```python
from build123d import *

# Parameters (mm, degrees)
BOSS_EXTRUDE1_DEPTH = 16.4
SKETCH3_R           = 4.85
CUT_EXTRUDE1_DEPTH  = 55.101495482


with BuildPart() as part:
    # Sketch1 → Revolve1 (revolve)
    with BuildSketch(Plane.XY, mode=Mode.PRIVATE) as revolve1_sk:
        Polygon((0, 51.4), (0, 0), (10.9, 0), (10.9, 3.8), (11.05, 3.8), (11.05, 20.1), (10.9, 20.1), (10.9, 22.1), (7.9, 22.1), (7.9, 24.4), (6.35, 24.4), (6.35, 34.8), (7.95, 34.8), (6.35, 39.6), (6.35, 44.2), (7.55, 44.2), (6.35, 48.4), (6.35, 51.4), align=None)
    revolve(revolve1_sk.sketch.rotate(Axis((0, 51.4, 0), (0, -1, 0)), 180), axis=Axis((0, 51.4, 0), (0, -1, 0)))

    # Sketch2 → Boss-Extrude1 (add)
    with BuildSketch(Plane(origin=(0, 20.1, 0), x_dir=(1, 0, 0), z_dir=(0, 1, 0))):
        Polygon((12.761813873, 0), (6.380906937, 11.052055013), (-6.380906937, 11.052055013), (-12.761813873, 0), (-6.380906937, -11.052055013), (6.380906937, -11.052055013), align=None)
    extrude(amount=-BOSS_EXTRUDE1_DEPTH)

    # Sketch3 → Cut-Extrude1 (cut, through all)
    with BuildSketch(Plane(origin=(0, 51.4, 0), x_dir=(1, 0, 0), z_dir=(0, 1, 0))):
        with Locations(Location((0, 0, 0), (0, 0, 180))):
            Circle(SKETCH3_R)
    extrude(amount=-CUT_EXTRUDE1_DEPTH, mode=Mode.SUBTRACT)


solid = part.part
```
For this review, take the finished solid that the model builds, in its own axes (mm). A direction names the side the tool comes from. Give positions to 0.01 mm unless a question says otherwise; leave off trailing zeros. Write each loop counter-clockwise with the first axis right and the second up, starting at its lowest first coordinate (ties: lowest second). Pieces come first, ordered by that corner, then holes. Notation, with made-up numbers: M 35,77.5 L 85,77.5 A11 cw 85,86.5 Z; hole C 10.5,73 d10. An arc over 180 degrees is marked long. Answer as CSV lines item,"result".
1. Draft analysis for pull direction Y (two halves, no side actions). For faces 5 (the flat face through (5, 0, 2)), 6 (the cylindrical face through (-5.03, 21.11, 9.67)), 7 (the conical face through (1.393, 39.367, 6.275)), 8 (the cylindrical face through (5.82, 23.27, -5.34)), state which applies: +Y half, -Y half, draft (parallel to the pull), parting line (faces both ways), or undercut.
Findings:
face 5,"-Y half"
face 6,"draft"
face 7,"undercut"
face 8,"undercut"
2. For faces 1 (the flat face through (11.3, 3.7, -0.1)), 2 (the cylindrical face through (-2.93, 49.921, 5.634)), 3 (the cylindrical face through (-2.93, 29.673, 5.634)), 4 (the flat face through (9.53, 12.01, 5.6)), list the 3-axis set-ups (+Z, -Z, +X, -X, +Y, -Y) from which the entire face can be reached by the end or side of a thin tool; tool diameter is ignored.
Findings:
face 1,"-Y"
face 2,"+Y"
face 3,"none"
face 4,"+Z, +X, +Y, -Y"
3. Consider section D-D, the plane z = 9.75. Write out the cut boundary in (x, y), then the cut area to 3 significant figures.
Findings:
outline,"M -7.13,3.7 L -4.87,3.7 L -4.87,0 L 4.87,0 L 4.87,3.7 L 7.13,3.7 L 7.13,20.1 L 4.87,20.1 L 4.87,22.1 L -4.87,22.1 L -4.87,20.1 L -7.13,20.1 Z"
area,"290 mm2"
4. Wall thickness on line 1 (Z direction, x = 0, y = 22); line 2 (Z direction, x = 0, y = 39.5); line 3 (Y direction, x = 0.75, z = -9.75): over which ranges is each line inside the solid? List them lowest first.
Findings:
line 1,"z = -10.9 to -4.85, 4.85 to 10.9"
line 2,"z = -6.38 to -4.85, 4.85 to 6.38"
line 3,"y = 0 to 22.1"
5. For pin 1 (10 mm diameter, centred on x = 6.5, z = 1.5, fed in from -Y); pin 2 (12 mm diameter, centred on x = -2, y = 30, fed in from -Z); pin 3 (1 mm diameter, centred on x = -1, y = 41.5, fed in from +Z); pin 4 (4 mm diameter, centred on x = -1, y = 22.5, fed in from -Z), all flat-tipped, find the tip position at first contact; note any pin that passes through.
Findings:
pin 1,"stops at y = 0"
pin 2,"stops at z = -7.95"
pin 3,"stops at z = 6.33"
pin 4,"stops at z = -10.9"
6. Consider section C-C, the plane x = -10. Write out the cut boundary in (y, z), then the cut area to 3 significant figures.
Findings:
outline,"M 0,-4.34 L 3.7,-4.34 L 3.7,-4.78 L 20.1,-4.78 L 20.1,-4.34 L 22.1,-4.34 L 22.1,4.34 L 20.1,4.34 L 20.1,4.78 L 3.7,4.78 L 3.7,4.34 L 0,4.34 Z"
area,"206 mm2"
7. Consider section A-A, the plane y = 12.5. Write out the cut boundary in (x, z).
Findings:
outline,"M -12.76,0 L -6.38,-11.05 L 6.38,-11.05 L 12.76,0 L 6.38,11.05 L -6.38,11.05 Z; hole C 0,0 d9.7"
8. Consider section B-B, the plane z = -7. Count the separate pieces of the cut face and the enclosed holes in it, then the cut area to 3 significant figures.
Findings:
separate pieces,"3"
enclosed holes,"0"
area,"419 mm2"
